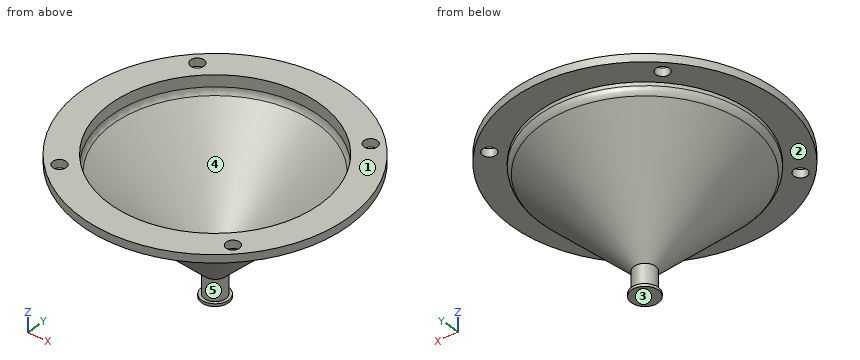
```python
from build123d import *

# Parameters (mm, degrees)
F0_R      = 250
F0_R_2    = 200
F1_DEPTH  = 15
F5_R      = 20
F6_DEPTH  = 40
F7_R      = 25.25
F8_DEPTH  = 5
F9_R      = 12.5
F10_DEPTH = 15


with BuildPart() as f1:
    # F0 (on Top) → F1 (new body)
    with BuildSketch(Plane.XY):
        Circle(F0_R)
        Circle(F0_R_2, mode=Mode.SUBTRACT)
    extrude(amount=F1_DEPTH)

    # F2 (on Front) → F3 (revolve)
    with BuildSketch(Plane.XZ):
        with BuildLine():
            Line((200, -6.715729), (200, 15))
            Line((200, 15), (197, 15))
            Line((197, 15), (197, -6.715729))
            ThreePointArc((197, -6.715729), (195.705952, -13.221347), (192.020815, -18.736544))
            Line((192.020815, -18.736544), (18.757359, -192))
            Line((18.757359, -192), (0, -192))
            Line((0, -192), (0, -195))
            Line((0, -195), (20, -195))
            Line((20, -195), (194.142136, -20.857864))
            ThreePointArc((194.142136, -20.857864), (198.477591, -14.369397), (200, -6.715729))
        make_face()
    revolve(axis=Axis((0, 0, -193.5), (0, 0, -1)))

    # F5 (on face) → F6 (join)
    with BuildSketch(Plane(origin=(0, 0, -195), x_dir=(1, 0, 0), z_dir=(0, 0, -1))):
        Circle(F5_R)
    extrude(amount=F6_DEPTH)

    # F7 (on face) → F8 (join)
    with BuildSketch(Plane(origin=(0, 0, -235), x_dir=(1, 0, 0), z_dir=(0, 0, -1))):
        Circle(F7_R)
    extrude(amount=F8_DEPTH)

    # F9 (on face) → F10 (cut)
    with BuildSketch(Plane.XY.offset(15)):
        with Locations((160.866793, 160.866793)):
            Circle(F9_R)
        with Locations((-160.866793, 160.866793)):
            Circle(F9_R)
        with Locations((-160.866793, -160.866793)):
            Circle(F9_R)
        with Locations((160.866793, -160.866793)):
            Circle(F9_R)
    extrude(amount=-F10_DEPTH, mode=Mode.SUBTRACT)


solid = f1.part
```
Here's how the part is built. I have some questions about the finished solid (model axes, mm). Face numbers are marked on the shaded views. A direction names the side the tool comes from. Give positions to 0.01 mm unless a question says otherwise; leave off trailing zeros. Write each loop counter-clockwise with the first axis right and the second up, starting at its lowest first coordinate (ties: lowest second). Pieces come first, ordered by that corner, then holes. Notation, with made-up numbers: M 58.5,84 L 94.5,84 A15 cw 94.5,102 Z; hole C -40,-39 d6. An arc over 180 degrees is marked long. Put each result on its own line as item: value. Start each with the question number.
Item 1: If we section it at D-D, the plane z = -148.5: Write out the boundary of the cut face in (x, y), then the cut area to 3 significant figures.
Item 2: Will these pins go through, and if not, where does the flat tip stop? pin 1 (12 mm diameter, centred on y = -32, z = -14, fed in from +X); pin 2 (15 mm diameter, centred on x = 160.87, y = -160.87, fed in from -Z); pin 3 (1 mm diameter, centred on x = 100.5, z = -70.5, fed in from +Y); pin 4 (12 mm diameter, centred on y = -26, z = -175, fed in from -X).
Item 3: If we section it at A-A, the plane y = 0: Write out the boundary of the cut face in (x, z).
Item 4: If we section it at C-C, the plane z = -105: Write out the boundary of the cut face in (x, y).
Item 5: I need wall thicknesses on L1, parallel to X at y = 0, z = -2; L2, parallel to X at y = 165.5, z = 4; L3, parallel to Z at x = 180.5, y = -97.5. Which ranges of each line are inside material? Lowest first, please. Write a range as from..to.
Item 6: Thinking about a two-plate mould opening in X: for the marked faces 3, 4 and 5, which applies, +X half, -X half, draft (parallel to the pull), parting line (faces both ways), or undercut?
Item 7: On a 3-axis mill with a long thin cutter (end or side, diameter ignored), from which of +Z, -Z, +X, -X, +Y, -Y can I reach the whole of each face in a straight line? I mean the marked faces 1 and 2. Say none if no direction works.
Values:
1. outline: C 0,0 d133; hole C 0,0 d124.51
1. area: 1,720 mm²
2. pin 1: x = 197.83
2. pin 2: through
2. pin 3: y = 104.67
2. pin 4: x = -38.92
3. outline: M -250,0 L -200,0 L -200,-6.72 A20 ccw -194.14,-20.86 L -20,-195 L -20,-235 L -25.25,-235 L -25.25,-240 L 25.25,-240 L 25.25,-235 L 20,-235 L 20,-195 L 194.14,-20.86 A20 ccw 200,-6.72 L 200,0 L 250,0 L 250,15 L 197,15 L 197,-6.72 A17 cw 192.02,-18.74 L 18.76,-192 L -18.76,-192 L -192.02,-18.74 A17 cw -197,-6.72 L -197,15 L -250,15 Z
4. outline: C 0,0 d220; hole C 0,0 d211.51
5. L1: -200..-197, 197..200
5. L2: -187.38..-172.48, -149.26..-106.86, 106.86..149.26, 172.48..187.38
5. L3: 0..15
6. face 3: draft
6. face 4: undercut
6. face 5: parting line
7. face 1: +Z, +X, -X, +Y, -Y
7. face 2: -Z
